Source: CAD feature listing. Evaluate the final solid. Frame: model axes, mm. A direction names the side the tool comes from. Round coordinates to 2 decimals unless told otherwise and drop trailing zeros. Order: outer loops, then holes, each group sorted by start corner. A loop starts at its lowest first (then second) coordinate and runs counter-clockwise, first axis right, second up. Notation, with made-up numbers: (50.5, 67) - (68.5, 67) arc R19 cw to (68.5, 71) - close; hole circle Ø8 at (13.5, 87.5). An arc over 180 degrees is marked (long way). Return JSON: item names as keys, results as strings. Group by question number.
1) Access query for faces 1 (the cylindrical face through (-28, 21, 22)), 2 (the flat face through (32.148, 19.318, 7.395)), 3 (the flat face through (6, -3, 31)). Directions: +Z, -Z, +X, -X, +Y, -Y. A direction counts if a zero-diameter tool reaches every point of the face in a straight line with its end or side. Return the directions, or none.
2) Section C-C, the plane x = 0. Give the number of separate pieces and of enclosed holes in the cut face, plus the area to 3 significant figures.
3) Contact query for flat-ended pins moving along their axis: P1, Ø11, axis at x = 0, y = 0, coming from the -Z side; P2, Ø3, axis at x = 35.5, y = 7.5, coming from the +Z side; P3, Ø4, axis at x = -8.5, z = 26.5, coming from the -Y side; P4, Ø8, axis at y = -7.5, z = 9, coming from the +X side. Output: stop coordinate, or through.
4) Section A-A, the plane y = 47.5. Return loops of the section in (x, z), plus the area to 3 significant figures.
5) Mould query, pull axis Y, two halves, no side actions, for faces 4 (the cylindrical face through (26.36, -5.85, 5.07)), 5 (the cylindrical face through (0, 60, 7)), 6 (the cylindrical face through (15.24, 6.32, 36.47)). Classes: pulls with the +Y half, pulls with the -Y half, needs draft (parallel to the pull), parting line crosses it, or undercut.
6) Section B-B, the plane z = 60.5. Return loops of the section in (x, y), plus the area to 3 significant figures.
7) Ray query, line 1 (Y direction, x = 0, z = 9.25); line 2 (X direction, y = 0, z = 52.5). Return the intervals inside material, ascending. Write a range as from..to.
Autodesk Inventor part; units mm, degrees
ref_plane "YZ Plane" through (0, 0, 0) normal (1, 0, 0) x (0, 1, 0)
ref_plane "XZ Plane" through (0, 0, 0) normal (0, 1, 0) x (-1, 0, 0)
ref_plane "XY Plane" through (0, 0, 0) normal (0, 0, 1) x (1, 0, 0)
sketch "Эскиз1" plane through (0, 0, 0) normal (0, 0, 1) x (1, 0, 0)
  line L0 (9.0572, 59.3125) -> (55.8947, -21.8125)
  line L1 (46.8375, -37.5) -> (-46.8375, -37.5)
  line L2 (-55.8947, -21.8125) -> (-9.0572, 59.3125)
  arc A0 (9.0572, 59.3125) -> (-9.0572, 59.3125) centre (0, 0) ccw
  arc A1 (-55.8947, -21.8125) -> (-46.8375, -37.5) centre (0, 0) ccw
  arc A2 (46.8375, -37.5) -> (55.8947, -21.8125) centre (0, 0) ccw
  circle A3 centre (0, 47.5) radius 6
  circle A4 centre (-41.1362, -23.75) radius 6
  circle A5 centre (41.1362, -23.75) radius 6
  dimension "d3" = 12
  dimension "d6" = 360
extrude "Выдавливание1" add sketch "Эскиз1" along normal blind 15
sketch "Эскиз2" plane through (0, 0, 15) normal (0, 0, 1) x (1, 0, 0)
  circle A0 centre (0, 0) radius 35
  dimension "d10" = 70
extrude "Выдавливание2" add sketch "Эскиз2" along normal blind 19
sketch "Эскиз3" plane through (0, 0, 0) normal (1, 0, 0) x (0, 1, 0)
  line L0 (-35, 15) -> (-35, 34)
  line L1 (35, 34) -> (-35, 34)
  line L2 (35, 15) -> (35, 34)
  line L3 (35, 29.3369) -> (25, 34)
  line L4 (0, 34) -> (0, 40.7436)
  point P0 (0, 0)
  dimension "d13" = 25
  dimension "d14" = 25
revolve "Вращение1" cut sketch "Эскиз3" angle 360 about axis through (0, 0, 34) along (0, 0, 1)
sketch "Эскиз4" plane through (0, 0, 34) normal (0, 0, 1) x (1, 0, 0)
  circle A0 centre (0, 0) radius 16.5
  dimension "d16" = 33
extrude "Выдавливание3" add sketch "Эскиз4" along normal blind 5
sketch "Эскиз5" plane through (0, 0, 39) normal (0, 0, 1) x (1, 0, 0)
  circle A0 centre (0, 0) radius 13.5
  dimension "d19" = 27
extrude "Выдавливание4" add sketch "Эскиз5" along normal blind 31
sketch "Эскиз6" plane through (0, 0, 0) normal (1, 0, 0) x (0, 1, 0)
  line L0 (-13.5, 39) -> (13.5, 39)
  line L1 (16.5, 39) -> (-16.5, 39)
  line L2 (13.5, 70) -> (-13.5, 70)
  line L3 (0, 70) -> (0, 78.8813)
  line L4 (12.1787, 39) -> (12.1787, 45)
  line L5 (12.1787, 45) -> (13.5, 46.3213)
  line L6 (13.5, 39) -> (13.5, 70)
  point P0 (0, 0)
  dimension "d22" = 45
  dimension "d23" = 6
revolve "Вращение2" cut sketch "Эскиз6" angle 360 about axis through (0, 0, 70) along (0, 0, 1)
fillet "Сопряжение1" radius 1.6 1 edges at (0, -12.1787, 39)
fillet "Сопряжение2" radius 1 1 edges at (0, -12.1787, 45)
thread "Резьба1"
chamfer "Фаска1" distance 2.5 angle 45 1 edges at (-13.5, 0, 70)
sketch "Эскиз7" plane through (0, 0, 0) normal (0, 0, -1) x (-1, 0, 0)
  point P0 (0, 0)
  point P1 (0, 0)
hole "Отверстие1" at (0, 0, 0) direction (0, 0, 1) diameter 54 depth 10
sketch "Эскиз8" plane through (0, 0, 10) normal (0, 0, -1) x (-1, 0, 0)
  point P0 (0, 0)
  point P1 (0, 0)
sketch "Эскиз9" plane through (0, 0, 70) normal (0, 0, 1) x (1, 0, 0)
  point P0 (0, 0)
  point P1 (0, 0)
hole "Отверстие2" at (0, 0, 70) direction (0, 0, -1) diameter 12 depth 39
chamfer "Фаска2" distance 1 angle 45 1 edges at (0, 6, 70)
sketch "Эскиз10" plane through (0, 0, 31) normal (0, 0, 1) x (1, 0, 0)
  point P0 (0, 0)
  point P1 (0, 0)
hole "Отверстие3" at (0, 0, 31) direction (0, 0, -1) diameter 28 end through all
sketch "Эскиз11" plane through (0, 0, 0) normal (1, 0, 0) x (0, 1, 0)
  line L0 (14, 10) -> (-14, 10)
  line L1 (-27, 10) -> (27, 10)
  line L2 (-14, 31) -> (14, 31)
  line L3 (0, 10) -> (0, -15.8706)
  line L4 (20, 10) -> (14, 16)
  line L5 (14, 10) -> (-14, 10)
  line L6 (-14, 31) -> (14, 31)
  line L7 (14, 10) -> (14, 22.3316)
  line L8 (14, 10) -> (14, 31)
  point P0 (0, 0)
  dimension "d56" = 45
  dimension "d57" = 6
revolve "Вращение3" cut sketch "Эскиз11" angle 360 about axis through (0, 0, 10) along (0, 0, -1)
properties part number "Люляев"
Geometry check:
{
 "1": {"face 1": "+Z", "face 2": "+Z, -Z, +X, +Y", "face 3": "-Z"},
 "2": {"separate pieces": "3", "enclosed holes": "0", "area": "1,910 mm2"},
 "3": {"P1": "through", "P2": "z = 29.44", "P3": "y = -34.39", "P4": "x = 49.94"},
 "4": {"outline": "(-15.88, 0) - (-6, 0) - (-6, 15) - (-15.88, 15) - close; (6, 0) - (15.88, 0) - (15.88, 15) - (6, 15) - close", "area": "296 mm2"},
 "5": {"face 4": "undercut", "face 5": "pulls with the +Y half", "face 6": "parting line crosses it"},
 "6": {"outline": "circle Ø27 at (0, 0); hole circle Ø12 at (0, 0)", "area": "459 mm2"},
 "7": {"line 1": "-37.5..-27, 27..41.5, 53.5..60", "line 2": "-13.5..-6, 6..13.5"}
}
